The listing builds one solid part. Answer for the finished solid, in the listing's coordinates (mm). Give positions to 0.01 mm unless a question says otherwise; leave off trailing zeros. Order: outer loops, then holes, each group sorted by start corner. A loop starts at its lowest first (then second) coordinate and runs counter-clockwise, first axis right, second up. Notation, with made-up numbers: (-6, 22.25) - (28, 22.25) arc R20 ccw to (28, 50.25) - close; hole circle Ø1 at (-35, 62). An arc over 180 degrees is marked (long way). Answer in a Markdown table with one row per item. Add a question column.
```python
from build123d import *

# Parameters (mm, degrees)
F1_DEPTH = 0.585


with BuildPart() as f1:
    # F0 (on Front) → F1 (new body, symmetric)
    with BuildSketch(Plane.XZ):
        with BuildLine():
            add(Edge.make_bspline(
                [(-0.9, 0), (-0.9, 3.8525), (0.05, 3.8525), (0.05, 7.705)],
                knots=[0, 0, 0, 0, 7.763345, 7.763345, 7.763345, 7.763345], degree=3))
            Line((-0.9, 0), (-0.9, -13.695881))
            Line((-0.9, -13.695881), (-0.9, -68.63))
            ThreePointArc((-0.9, -68.63), (-1.55901, -70.22099), (-3.15, -70.88))
            Line((-3.15, -70.88), (-14.135, -70.88))
            ThreePointArc((-14.135, -70.88), (-15.99, -72.735), (-14.135, -74.59))
            Line((-14.135, -74.59), (-3.15, -74.59))
            ThreePointArc((-3.15, -74.59), (-1.55901, -75.24901), (-0.9, -76.84))
            Line((-0.9, -76.84), (-0.9, -126.99))
            ThreePointArc((-0.9, -126.99), (0, -127.89), (0.9, -126.99))
            Line((0.9, -126.99), (0.9, -76.84))
            ThreePointArc((0.9, -76.84), (-0.286218, -73.976218), (-3.15, -72.79))
            Line((-3.15, -72.79), (-14.135, -72.79))
            ThreePointArc((-14.135, -72.79), (-14.19, -72.735), (-14.135, -72.68))
            Line((-14.135, -72.68), (-3.15, -72.68))
            ThreePointArc((-3.15, -72.68), (-0.286218, -71.493782), (0.9, -68.63))
            Line((0.9, -68.63), (0.9, -13.775932))
            Line((0.9, -13.775932), (0.9, 0))
            Line((0.9, 0), (0.9, 7.705))
            ThreePointArc((0.9, 7.705), (-0.785, 9.39), (-2.47, 7.705))
            ThreePointArc((-2.47, 7.705), (-2.045, 7.28), (-1.62, 7.705))
            ThreePointArc((-1.62, 7.705), (-0.785, 8.54), (0.05, 7.705))
        make_face()
    extrude(amount=F1_DEPTH, both=True)


solid = f1.part
```
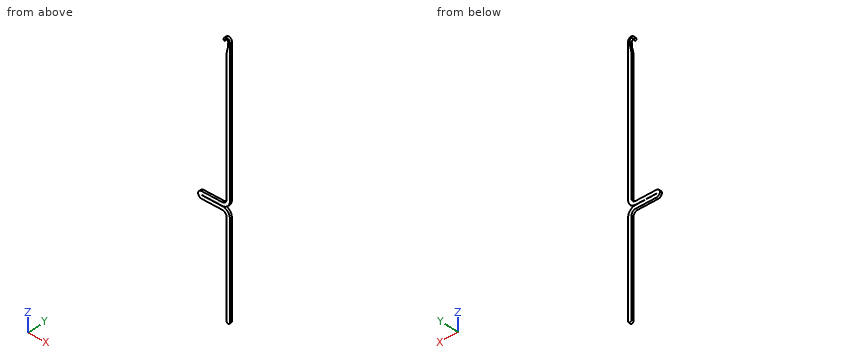
(1) Find section B-B, the plane z = -40.5. Write down the section's boundary in (x, y) (3 decimals), plus the area to 3 significant figures.
(2) Find section A-A, the plane x = -11.25. Write down the section's boundary in (y, z) (3 decimals).
(3) Straight lines are drawn through the part: line 1 (Z direction, x = -1.5, y = 0.2); line 2 (X direction, y = 0.55, z = -46); line 3 (Z direction, x = -2.75, y = -0.4). For each, find the intervals that lie inside material, in ascending order.
(4) This flat-tipped pin is pushed along its axis until it touches: P1, Ø0.6, axis at y = 0, z = -105.5, coming from the -X side. Where does it stop, or does it pass through?
Answer key:
| question | item | result |
|---|---|---|
| 1 | outline | (-0.9, -0.585) - (0.9, -0.585) - (0.9, 0.585) - (-0.9, 0.585) - close |
| 1 | area | 2.11 mm² |
| 2 | outline | (-0.585, -74.59) - (0.585, -74.59) - (0.585, -72.79) - (-0.585, -72.79) - close; (-0.585, -72.68) - (0.585, -72.68) - (0.585, -70.88) - (-0.585, -70.88) - close |
| 3 | line 1 | -75.31 to -73.14, -72.33 to -70.16, 8.14 to 9.23 |
| 3 | line 2 | -0.9 to 0.9 |
| 3 | line 3 | -74.63 to -72.81, -72.66 to -70.84 |
| 4 | P1 | x = -0.9 |
